CAD build for the part. Positions are in the model's coordinates, mm. A direction names the side the tool comes from. Coordinates: 2 decimals unless noted, no trailing zeros. Loops run counter-clockwise (first coordinate to the right, second up) from the corner with the lowest first, then second, coordinate; pieces in that order, holes last. Notation, with made-up numbers: (13, 76.5) -> (51, 76.5) arc R25 cw to (51, 104.5) -> close; hole circle Ø3 at (-15.5, 62.25). An arc over 180 degrees is marked (long way). Write each question's results on one line, items separated by ' | '.
```python
from build123d import *

# Parameters (mm, degrees)
F1_DEPTH  = 43
F2_R      = 4
F3_DEPTH  = 6
F4_R      = 1.5
F5_DEPTH  = 25
F4_R_2    = 3
F6_DEPTH  = 1.5
F7_W      = 10
F7_H      = 4.5
F8_DEPTH  = 5
F10_DEPTH = 50
F11_R     = 2
F13_R     = 1.35
F14_DEPTH = 12


with BuildPart() as f1:
    # F0 (on Front) → F1 (new body, symmetric)
    with BuildSketch(Plane.XZ):
        with BuildLine():
            Line((0, 11.5), (0, 69))
            Line((0, 69), (-5, 69))
            Line((-5, 69), (-5, 0))
            Line((-5, 0), (23, 0))
            Line((23, 0), (23, 13))
            Line((23, 13), (20, 13))
            Line((20, 13), (18, 11))
            Line((18, 11), (0.5, 11))
            ThreePointArc((0.5, 11), (0.146447, 11.146447), (0, 11.5))
        make_face()
    extrude(amount=F1_DEPTH, both=True)

    # F2 (on face) → F3 (cut)
    with BuildSketch(Plane(origin=(0, 0, 0), x_dir=(1, 0, 0), z_dir=(0, 0, -1))):
        with Locations((3, -33)):
            Circle(F2_R)
        with Locations((3, -8)):
            Circle(F2_R)
        with Locations((3, 32)):
            Circle(F2_R)
    extrude(amount=-F3_DEPTH, mode=Mode.SUBTRACT)

    # F4 (on face) → F5 (cut)
    with BuildSketch(Plane.XY.offset(11)):
        with Locations((3, 33)):
            Circle(F4_R)
        with Locations((3, 8)):
            Circle(F4_R)
        with Locations((3, -32)):
            Circle(F4_R)
    extrude(amount=-F5_DEPTH, mode=Mode.SUBTRACT)

    # F4 (on face) → F6 (cut, symmetric)
    with BuildSketch(Plane.XY.offset(11)):
        with Locations((3, 8)):
            Circle(F4_R_2)
        with Locations((3, 8)):
            Circle(F4_R, mode=Mode.SUBTRACT)
        with Locations((3, 33)):
            Circle(F4_R_2)
        with Locations((3, 33)):
            Circle(F4_R, mode=Mode.SUBTRACT)
        with Locations((3, -32)):
            Circle(F4_R_2)
        with Locations((3, -32)):
            Circle(F4_R, mode=Mode.SUBTRACT)
    extrude(amount=F6_DEPTH, both=True, mode=Mode.SUBTRACT)

    # F7 (on face) → F8 (join)
    with BuildSketch(Plane.XY.offset(11)):
        with Locations((10, 40.75)):
            Rectangle(F7_W, F7_H)
        with Locations((10, -20.75)):
            Rectangle(F7_W, F7_H)
    extrude(amount=F8_DEPTH)

    # F9 (on Front) → F10 (cut, symmetric)
    with BuildSketch(Plane.XZ):
        Polygon((5, 19), (5, 11), (13, 19), align=None)
    extrude(amount=F10_DEPTH, both=True, mode=Mode.SUBTRACT)

    # F11
    f11_edges = [f1.edges().sort_by_distance(p)[0] for p in [
        (23, -43, 6.5),
        (23, 43, 6.5),
        (-2.5, -43, 69),
        (-2.5, 43, 69),
    ]]
    fillet(f11_edges, radius=F11_R)

    # F13 (on face) → F14 (cut)
    with BuildSketch(Plane.XY.offset(69)):
        with Locations((-2.5, -18)):
            Circle(F13_R)
    extrude(amount=-F14_DEPTH, mode=Mode.SUBTRACT)


solid = f1.part
```
Q1. Which spindle directions (+Z, -Z, +X, -X, +Y, -Y) get a long thin tool onto all of the face, cutting with end or side? Do faces 5 (the flat face through (7, 41, 13)), 6 (the flat face through (3, 35, 6)), 7 (the flat face through (4.3, 6.7, 9.5)), 8 (the cylindrical face through (22.43, 42.4, 6.59)). Say none if no direction does.
Results are:
face 5: +Z, +Y, -Y | face 6: -Z | face 7: +Z | face 8: +Z, -Z, +X, +Y
Q2. Pull direction X, two halves, no side cores. Call faces 1 (the cylindrical face through (-2.54, -42.43, 68.4)), 2 (the flat face through (4.3, 31.7, 9.5)), 3 (the flat face through (19, -1, 12)), 4 (the flat face through (-5, -1, 35)): +X half, -X half, draft (parallel to the pull), parting line (faces both ways), or undercut.
Results are:
face 1: draft | face 2: undercut | face 3: undercut | face 4: -X half
Q3. Cut at B-B on x = 8.5. Write the cut outline in (y, z), and give its area (4 significant figures).
Results are:
outline: (-43, 0) -> (43, 0) -> (43, 14.5) -> (38.5, 14.5) -> (38.5, 11) -> (-18.5, 11) -> (-18.5, 14.5) -> (-23, 14.5) -> (-23, 11) -> (-43, 11) -> close | area: 977.5 mm^2
Q4. Cut at C-C on y = 27. Write the cut outline in (x, z).
Results are:
outline: (-5, 0) -> (23, 0) -> (23, 13) -> (20, 13) -> (18, 11) -> (0.5, 11) arc R0.5 cw to (0, 11.5) -> (0, 69) -> (-5, 69) -> close
Q5. Drop flat-ended pins along their axis: pin 1 (1.3 mm diameter, centred on x = 13, y = -20.5, fed in from +Z); pin 2 (9 mm diameter, centred on x = 9, y = -5.5, fed in from +Z); pin 3 (2 mm diameter, centred on y = 27.5, z = 58, fed in from +X). Give the stop position or say it passes through.
Results are:
pin 1: z = 16 | pin 2: z = 11 | pin 3: x = 0
Q6. Cut at A-A on z = 59.5. Write the cut outline in (x, y).
Results are:
outline: (-5, -43) -> (0, -43) -> (0, 43) -> (-5, 43) -> close; hole circle Ø2.7 at (-2.5, -18)
Q7. Cut at D-D on x = 3. Give the number of separate pieces and of enclosed holes in the cut face, and give its area (4 significant figures).
Results are:
separate pieces: 4 | enclosed holes: 0 | area: 743.5 mm^2
Q8. Wall check: L1, parallel to Y at x = 3, z = 10.65; L2, parallel to Y at x = 3, z = 2.45; L3, parallel to X at y = 8, z = 2. Give the ranges that are in metal, low to high. Write a range as from..to.
Results are:
L1: -43..-35, -29..5, 11..30, 36..43 | L2: -43..-36, -28..4, 12..29, 37..43 | L3: -5..-1, 7..23
